Here's how the part is built. I have some questions about the finished solid (model axes, mm). Face numbers are marked on the shaded views. A direction names the side the tool comes from. Coordinates: 2 decimals unless noted, no trailing zeros. Write each loop counter-clockwise with the first axis right and the second up, starting at its lowest first coordinate (ties: lowest second). Pieces come first, ordered by that corner, then holes. Notation, with made-up numbers: (-11.5, -25) -> (-3.5, -25) arc R32 ccw to (-3.5, 12) -> close; hole circle Ø4 at (-1.75, 66.5). An arc over 180 degrees is marked (long way). Put each result on its own line as item: value. Start each with the question number.
Item 1: I want a section at D-D, the plane y = 12. List the corners of the cut face in (x, z) for me, then the cut area to 3 significant figures.
Item 2: On a 3-axis mill with a long thin cutter (end or side, diameter ignored), from which of +Z, -Z, +X, -X, +Y, -Y can I reach the whole of each face in a straight line? I mean the marked faces 1 and 2. Say none if no direction works.
Item 3: I want a section at C-C, the plane y = 4. List the corners of the cut face in (x, z) for me.
Item 4: I need wall thicknesses on line 1 (X direction, y = -0.5, z = 8.5); line 2 (X direction, y = -6, z = 6.75); line 3 (Y direction, x = -10.25, z = 1.9). Which ranges of each line are inside material? Lowest first, please. Write a range as [from, to].
Item 5: I want a section at A-A, the plane x = 10.25. List the corners of the cut face in (y, z) for me.
Item 6: If we mould it in two halves opening along Y, with no side actions, what happens to the marked faces 3, 4 and 5? For each: released by +Y, released by -Y, zero draft, split by the parting line, or undercut.
Item 7: I want a section at B-B, the plane z = 12. List the corners of the cut face in (x, y) for me (3 decimals).
Item 8: For pin 1 (5 mm diameter, centred on x = -10.25, y = 0, fed in from -Z); pin 2 (8 mm diameter, centred on y = 4, z = 10.5, fed in from +X); pin 3 (2 mm diameter, centred on x = -9.5, y = 0, fed in from -Z); pin 4 (2.5 mm diameter, centred on x = 10.25, y = 0, fed in from -Z), each with a flat end and sliding along its axis, tell me the tip position at first contact or that it passes through.
from build123d import *

# Parameters (mm, degrees)
SKETCH_1_R               = 15.75
EXTRUDE_1_DEPTH          = 5.5
SKETCH_3_R               = 15.05
EXTRUDE_2_DEPTH          = 8
SKETCH_4_R               = 1.6
CUT_EXTRUDE_2_DEPTH      = 14.5
SKETCH_5_R               = 2.15
CUT_EXTRUDE_3_DEPTH      = 11.5
SKETCH_8_R               = 3.5
CUT_EXTRUDE_7_DEPTH      = 5.5
PATTERN_CIRCULAR_2_COUNT = 6
SKETCH_6_R               = 6.5
CUT_EXTRUDE_4_DEPTH      = 14.5
SKETCH_7_R               = 7.55
CUT_EXTRUDE_5_DEPTH      = 4
SKETCH_2_R               = 1.55
CUT_EXTRUDE_6_DEPTH      = 7
SKETCH_9_W               = 1.33041347
SKETCH_9_H               = 3
CUT_EXTRUDE_8_DEPTH      = 7
PATTERN_CIRCULAR_3_COUNT = 6


with BuildPart() as part:
    # 草图1 → 凸台-拉伸1 (new body)
    with BuildSketch(Plane.XY):
        Circle(SKETCH_1_R)
    extrude(amount=EXTRUDE_1_DEPTH)

    # 草图3 → 凸台-拉伸2 (add)
    with BuildSketch(Plane.XY.offset(5.5)):
        Circle(SKETCH_3_R)
    extrude(amount=EXTRUDE_2_DEPTH)

    # 草图4 → 切除-拉伸2 (cut, through all)
    with BuildSketch(Plane(origin=(0, 0, 0), x_dir=(-1, 0, 0), z_dir=(0, 0, -1))):
        with Locations((-10.25, 0)):
            Circle(SKETCH_4_R)
    cut_extrude_2 = extrude(amount=-CUT_EXTRUDE_2_DEPTH, mode=Mode.SUBTRACT)

    # 草图5 → 切除-拉伸3 (cut)
    with BuildSketch(Plane(origin=(0, 0, 0), x_dir=(-1, 0, 0), z_dir=(0, 0, -1))):
        with Locations((-10.25, 0)):
            Circle(SKETCH_5_R)
    cut_extrude_3 = extrude(amount=-CUT_EXTRUDE_3_DEPTH, mode=Mode.SUBTRACT)

    # 草图8 → 切除-拉伸7 (cut)
    with BuildSketch(Plane(origin=(0, 0, 0), x_dir=(-1, 0, 0), z_dir=(0, 0, -1))):
        with Locations((-10.25, 0)):
            Circle(SKETCH_8_R)
    cut_extrude_7 = extrude(amount=-CUT_EXTRUDE_7_DEPTH, mode=Mode.SUBTRACT)

    # 阵列(圆周)2: 切除-拉伸2, 切除-拉伸3, 切除-拉伸7 ×6 about axis
    pattern_circular_2_axis = Axis((0, 0, 0), (0, 0, 1))
    for i in range(1, PATTERN_CIRCULAR_2_COUNT):
        add(cut_extrude_2.rotate(pattern_circular_2_axis, i * 360 / PATTERN_CIRCULAR_2_COUNT), mode=Mode.SUBTRACT)
        add(cut_extrude_3.rotate(pattern_circular_2_axis, i * 360 / PATTERN_CIRCULAR_2_COUNT), mode=Mode.SUBTRACT)
        add(cut_extrude_7.rotate(pattern_circular_2_axis, i * 360 / PATTERN_CIRCULAR_2_COUNT), mode=Mode.SUBTRACT)

    # 草图6 → 切除-拉伸4 (cut, through all)
    with BuildSketch(Plane(origin=(0, 0, 0), x_dir=(-1, 0, 0), z_dir=(0, 0, -1))):
        Circle(SKETCH_6_R)
    extrude(amount=-CUT_EXTRUDE_4_DEPTH, mode=Mode.SUBTRACT)

    # 草图7 → 切除-拉伸5 (cut)
    with BuildSketch(Plane(origin=(0, 0, 0), x_dir=(-1, 0, 0), z_dir=(0, 0, -1))):
        Circle(SKETCH_7_R)
    extrude(amount=-CUT_EXTRUDE_5_DEPTH, mode=Mode.SUBTRACT)

    # 草图2 → 切除-拉伸6 (cut)
    with BuildSketch(Plane(origin=(0, 0, 0), x_dir=(-1, 0, 0), z_dir=(0, 0, -1))):
        with Locations((0, 12)):
            Circle(SKETCH_2_R)
    cut_extrude_6 = extrude(amount=-CUT_EXTRUDE_6_DEPTH, mode=Mode.SUBTRACT)

    # 草图9 → 切除-拉伸8 (cut)
    with BuildSketch(Plane(origin=(0, 0, 0), x_dir=(-1, 0, 0), z_dir=(0, 0, -1))):
        with Locations((0, 14.9)):
            Rectangle(SKETCH_9_W, SKETCH_9_H)
    cut_extrude_8 = extrude(amount=-CUT_EXTRUDE_8_DEPTH, mode=Mode.SUBTRACT)

    # 阵列(圆周)3: 切除-拉伸6, 切除-拉伸8 ×6 about axis
    pattern_circular_3_axis = Axis((0, 0, 0), (0, 0, 1))
    for i in range(1, PATTERN_CIRCULAR_3_COUNT):
        add(cut_extrude_6.rotate(pattern_circular_3_axis, i * 360 / PATTERN_CIRCULAR_3_COUNT), mode=Mode.SUBTRACT)
        add(cut_extrude_8.rotate(pattern_circular_3_axis, i * 360 / PATTERN_CIRCULAR_3_COUNT), mode=Mode.SUBTRACT)


solid = part.part
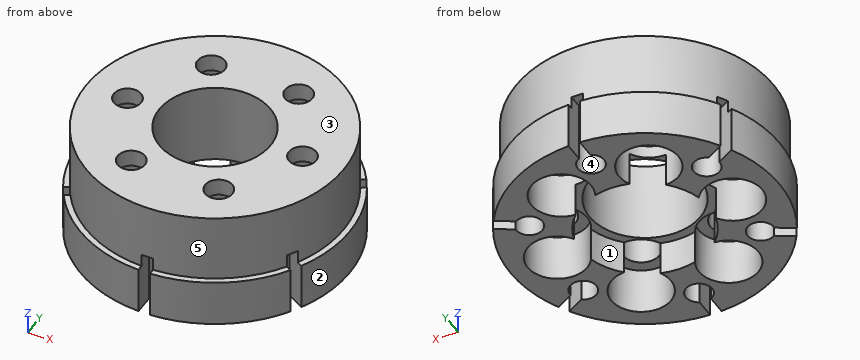
Calculated:
1. outline: (-10.2, 0) -> (-6.7, 0) -> (-6.7, 5.5) -> (-3.55, 5.5) -> (-3.55, 0) -> (-1.55, 0) -> (-1.55, 7) -> (1.55, 7) -> (1.55, 0) -> (3.55, 0) -> (3.55, 5.5) -> (6.7, 5.5) -> (6.7, 0) -> (10.2, 0) -> (10.2, 5.5) -> (9.08, 5.5) -> (9.08, 13.5) -> (-9.08, 13.5) -> (-9.08, 5.5) -> (-10.2, 5.5) -> close
1. area: 201 mm2
2. face 1: -Z
2. face 2: +Z, -Z, +X
3. outline: (-15.23, 0) -> (-6.4, 0) -> (-6.4, 4) -> (-5.12, 4) -> (-5.12, 13.5) -> (-14.51, 13.5) -> (-14.51, 5.5) -> (-15.23, 5.5) -> close; (5.12, 4) -> (6.4, 4) -> (6.4, 0) -> (15.23, 0) -> (15.23, 5.5) -> (14.51, 5.5) -> (14.51, 13.5) -> (5.12, 13.5) -> close
4. line 1: x = [-15.04, -12.34], [-8.16, -6.48], [6.48, 8.16], [12.34, 15.04]
4. line 2: x = [-13.8, -11.94], [-8.84, -2.5], [2.5, 8.84], [11.94, 13.8]
4. line 3: y = [-11.96, -7.54], [-4.46, -3.5], [3.5, 4.46], [7.54, 11.96]
5. outline: (-11.96, 0) -> (-7.54, 0) -> (-7.54, 7) -> (-4.46, 7) -> (-4.46, 0) -> (-3.5, 0) -> (-3.5, 5.5) -> (-2.15, 5.5) -> (-2.15, 11.5) -> (-1.6, 11.5) -> (-1.6, 13.5) -> (-11.02, 13.5) -> (-11.02, 5.5) -> (-11.96, 5.5) -> close; (1.6, 11.5) -> (2.15, 11.5) -> (2.15, 5.5) -> (3.5, 5.5) -> (3.5, 0) -> (4.46, 0) -> (4.46, 7) -> (7.54, 7) -> (7.54, 0) -> (11.96, 0) -> (11.96, 5.5) -> (11.02, 5.5) -> (11.02, 13.5) -> (1.6, 13.5) -> close
6. face 3: zero draft
6. face 4: undercut
6. face 5: split by the parting line
7. outline: circle Ø30.1 at (0, 0); hole circle Ø3.2 at (-10.25, 0); hole circle Ø3.2 at (-5.125, -8.877); hole circle Ø3.2 at (-5.125, 8.877); hole circle Ø13 at (0, 0); hole circle Ø3.2 at (5.125, -8.877); hole circle Ø3.2 at (5.125, 8.877); hole circle Ø3.2 at (10.25, 0)
8. pin 1: stops at z = 5.5
8. pin 2: stops at x = 15.05
8. pin 3: stops at z = 11.5
8. pin 4: passes through
